Could you check a few things on this model? Use its own coordinates, in mm. Round coordinates to 2 decimals unless told otherwise and drop trailing zeros. Loops run counter-clockwise (first coordinate to the right, second up) from the corner with the lowest first, then second, coordinate; pieces in that order, holes last. Notation, with made-up numbers: (28.5, 85) - (83.5, 85) arc R24 cw to (83.5, 117) - close; hole circle Ø7 at (78.5, -16). An arc over 180 degrees is marked (long way). Put each result on its own line as item: value. Start each with the question number.
from build123d import *


with BuildPart() as f1:
    # F0 (on Right) → F1 (revolve)
    with BuildSketch(Plane.YZ):
        with BuildLine():
            Line((0, 8), (0, 0))
            Line((0, 0), (102, 0))
            Line((102, 0), (102, 8))
            Line((102, 8), (65.41225, 8))
            ThreePointArc((65.41225, 8), (65.1, 7.85), (64.78775, 8))
            Line((64.78775, 8), (57.747999, 8))
            ThreePointArc((57.747999, 8), (55.25, 6.8), (52.752001, 8))
            Line((52.752001, 8), (0, 8))
        make_face()
    revolve(axis=Axis((0, 51, 0), (0, -1, 0)))


solid = f1.part
Item 1: Will these pins go through, and if not, where does the flat tip stop? P1, Ø4, axis at x = 6, z = 6, coming from the +Y side; P2, Ø1, axis at x = 3, y = 62, coming from the +Z side.
Item 2: Suppose I cut it at A-A, the plane y = 78. List the corners of the cut face in (x, z) for me, then the cut area to 3 significant figures.
Item 3: Thinking about a two-plate mould opening in Y: for faces 1 (the face through (0, 102, 0)), 2 (the face through (0, 0, 0)), 3 (the face through (7.81, 61.22, -1.73)), which applies, released by +Y, released by -Y, zero draft, split by the parting line, or undercut?
Item 4: I need wall thicknesses on line 1 (X direction, y = 52.5, z = -0.25); line 2 (Z direction, x = 6.75, y = 49.5); line 3 (Z direction, x = 3.75, y = 91.5). Which ranges of each line are inside material? Lowest first, please. Write a range as from..to.
Numbers:
1. P1: y = 102
1. P2: z = 7.6
2. outline: circle Ø16 at (0, 0)
2. area: 201 mm^2
3. face 1: released by +Y
3. face 2: released by -Y
3. face 3: zero draft
4. line 1: -8..8
4. line 2: -4.29..4.29
4. line 3: -7.07..7.07
